The listing builds one solid part. Answer for the finished solid, in the listing's coordinates (mm). Coordinates: 2 decimals unless noted, no trailing zeros. Order: outer loops, then holes, each group sorted by start corner. A loop starts at its lowest first (then second) coordinate and runs counter-clockwise, first axis right, second up. Notation, with made-up numbers: (-37, 74) - (11, 74) arc R10 ccw to (11, 82) - close; hole circle Ø7 at (41.25, 31.25). An arc over 180 degrees is marked (long way). Use one line per item in the form item = value. Start each with the question number.
Item 1: Consider line 1 along Z through (x, y) = (0, 0.8); line 2 along Z through (x, y) = (-9.25, 1.7); line 3 along X through (y, z) = (1.4, -12.25). Determine where each line is inside the solid, lowest interval first. Write a range as [from, to].
Item 2: This flat-tipped pin is pushed along its axis until it touches: pin 1 Ø2.5 at (x, z) = (-10.83, 6.25) entering from -Y. Where does it stop, or does it pass through?
Item 3: Section C-C, the plane y = 1.65 is taken. Write down the section's boundary in (x, z), and give its area (3 significant figures).
Item 4: The mould has two halves that part along X. Classify faces 1 (the flat face through (-9, 2, -5)), 2 (the cylindrical face through (-9.62, 0.99, 8.44)), 3 (the cylindrical face through (0, 1, -14)): released by +X, released by -X, zero draft, split by the parting line, or undercut.
Item 5: Section D-D, the plane x = -3.75 is taken. Write down the section's boundary in (y, z).
Item 6: Section B-B, the plane x = -11.5 is taken. Write down the section's boundary in (y, z), and give its area (3 significant figures).
Item 7: Section A-A, the plane z = 7.25 is taken. Write down the section's boundary in (x, y), and give its area (3 significant figures).
from build123d import *

# Parameters (mm, degrees)
SKETCH2_R           = 15
SKETCH2_R_2         = 10
SKETCH2_R_3         = 1.5
BOSS_EXTRUDE3_DEPTH = 2
CUT_EXTRUDE1_DEPTH  = 2
BOSS_EXTRUDE4_START = -2
SKETCH5_R           = 2.5
SKETCH5_R_2         = 1.5
BOSS_EXTRUDE4_DEPTH = 2


with BuildPart() as part:
    # Sketch2 → Boss-Extrude3 (new body)
    with BuildSketch(Plane(origin=(0, 0, 0), x_dir=(1, 0, 0), z_dir=(0, 1, 0))):
        with Locations(Location((0, 0, 0), (0, 0, 270))):
            Circle(SKETCH2_R)
        with Locations(Location((0, 0, 0), (0, 0, 270))):
            Circle(SKETCH2_R_2, mode=Mode.SUBTRACT)
        with Locations(Location((0, 12.5, 0), (0, 0, 270))):
            Circle(SKETCH2_R_3, mode=Mode.SUBTRACT)
        with Locations(Location((10.825317547, -6.25, 0), (0, 0, 270))):
            Circle(SKETCH2_R_3, mode=Mode.SUBTRACT)
        with Locations(Location((-10.825317547, -6.25, 0), (0, 0, 270))):
            Circle(SKETCH2_R_3, mode=Mode.SUBTRACT)
    extrude(amount=BOSS_EXTRUDE3_DEPTH)

    # Sketch4 → Cut-Extrude1 (cut)
    with BuildSketch(Plane(origin=(0, 2, 0), x_dir=(1, 0, 0), z_dir=(0, 1, 0))):
        Polygon((0, -17.282816366), (0, 0), (-10.825317547, -6.25), (-3.247954002, -19.374378648), (-1.635577826, -22.167096106), (6.824242843, -17.282816366), align=None)
        Polygon((9.189739722, -15.917096106), (0, 0), (0, -17.282816366), (6.824242843, -17.282816366), align=None)
        Polygon((0, 15), (0, 0), (9.189739722, -15.917096106), (6.824242843, -17.282816366), (15, -17.282816366), (15, 15), align=None)
        Polygon((-3.247954002, -19.374378648), (-10.825317547, -6.25), (-12.990381057, -7.5), (-5.413017511, -20.624378648), align=None)
    extrude(amount=-CUT_EXTRUDE1_DEPTH, mode=Mode.SUBTRACT)

    # Sketch5 → Boss-Extrude4 (add)
    # profile 1 of 2: a face of its own
    with BuildSketch(Plane(origin=(0, 2, 0), x_dir=(1, 0, 0), z_dir=(0, 1, 0)).offset(BOSS_EXTRUDE4_START)):
        with Locations((0, 12.5)):
            Circle(SKETCH5_R)
        with Locations(Location((0, 12.5, 0), (0, 0, 270))):
            Circle(SKETCH5_R_2, mode=Mode.SUBTRACT)
    # profile 2 of 2: a face of its own
    with BuildSketch(Plane(origin=(0, 2, 0), x_dir=(1, 0, 0), z_dir=(0, 1, 0)).offset(BOSS_EXTRUDE4_START)):
        with Locations((-10.825317547, -6.25)):
            Circle(SKETCH5_R)
        with Locations(Location((-10.825317547, -6.25, 0), (0, 0, 270))):
            Circle(SKETCH5_R_2, mode=Mode.SUBTRACT)
    extrude(amount=BOSS_EXTRUDE4_DEPTH)


solid = part.part
Response:
q1.line_1 = [-15, -14], [-11, -10]
q1.line_2 = [-11.81, -3.8], [3.8, 8.19]
q1.line_3 = [-8.66, -1.48], [1.48, 2.49]
q2.pin_1 = through
q3.outline = (-12.99, 7.5) arc R15 ccw to (0, -15) arc R2.5 ccw to (0, -10) arc R10 cw to (-8.66, 5) arc R2.5 ccw to start; hole circle Ø3 at (-10.83, 6.25); hole circle Ø3 at (0, -12.5)
q3.area = 136 mm2
q4.face_1 = zero draft
q4.face_2 = split by the parting line
q4.face_3 = undercut
q5.outline = (0, -14.52) - (2, -14.52) - (2, -9.27) - (0, -9.27) - close
q6.outline = (0, -9.63) - (2, -9.63) - (2, 4.91) - (0, 4.91) - close; (0, 7.59) - (2, 7.59) - (2, 8.66) - (0, 8.66) - close
q6.area = 31.2 mm2
q7.outline = (-13.13, 0) - (-11.94, 0) - (-11.94, 2) - (-13.13, 2) - close; (-9.71, 0) - (-8.53, 0) - (-8.53, 2) - (-9.71, 2) - close
q7.area = 4.72 mm2
